Work out the finished part from the listing and answer in its coordinate system (mm). Round coordinates to 2 decimals unless told otherwise and drop trailing zeros. Loops run counter-clockwise (first coordinate to the right, second up) from the corner with the lowest first, then second, coordinate; pieces in that order, holes last.
```python
from build123d import *

# Parameters (mm, degrees)
TD_STD_FEATURE_DEPTH            = 21.0312
ISA_STD_FEATURE_DEPTH           = 22.061040395498036
ISA_STD_FEATURE_DEPTH_BACK      = 22.061040395498036
BA_STD_FEATURE_DEPTH            = 22.061040395498036
BA_STD_FEATURE_DEPTH_BACK       = 22.061040395498036
VR_STD_FEATURE_DEPTH            = 22.061040395498036
VR_STD_FEATURE_DEPTH_BACK       = 22.061040395498036
ND_STD_FEATURE_DEPTH            = 22.061040395498036
ND_STD_FEATURE_DEPTH_BACK       = 22.061040395498036
HOLE_STD_FEATURE_D              = 0.381
HOLE_STD_FEATURE_CSINK_D        = 0.635
HOLE_STD_FEATURE_CSINK_ANGLE    = 60
STD_HOLE_CUT_FEATURE_DEPTH      = 22.158574025318714
STD_HOLE_CUT_FEATURE_DEPTH_BACK = 22.158574025318714
NR_FEATURE_R                    = 0.0254
STD_C_FEATURE_DEPTH             = 22.061040395498036
STD_C_FEATURE_DEPTH_BACK        = 22.061040395498036
STD_FR_C_FEATURE_R              = 0.01016
STD_BR_C_FEATURE_R              = 0.01016


with BuildPart() as part:
    # td_std_sketch → td_std_feature (new body)
    with BuildSketch(Plane(origin=(0, 0, 0), x_dir=(1, 0, 0), z_dir=(0, 1, 0))):
        with BuildLine():
            Line((-0.65532, 0.4456234374446657), (-0.6553199999999998, -0.44562343744466604))
            ThreePointArc((-0.6553199999999998, -0.44562343744466604), (0.79248, 0), (-0.65532, 0.4456234374446657))
        make_face()
    extrude(amount=TD_STD_FEATURE_DEPTH)

    # isa_std_sketch → isa_std_feature (cut, two sides: drawn at the far end of the back side and taken through both)
    with BuildSketch(Plane(origin=(0, 0, 0), x_dir=(0, 0, -1), z_dir=(1, 0, 0)).offset(-ISA_STD_FEATURE_DEPTH_BACK)):
        Polygon((8.373162888528082, 47.27049062508045), (0.79248, 4.278301579083286), (0.03809999999999999, 0), (-0.03809999999999999, 0), (-0.79248, 4.278301579083286), (-8.373162888528082, 47.27049062508045), (-8.373162888528082, -40.04033509597618), (8.373162888528082, -40.04033509597618), align=None)
    extrude(amount=ISA_STD_FEATURE_DEPTH + ISA_STD_FEATURE_DEPTH_BACK, mode=Mode.SUBTRACT)

    # ba_std_sketch → ba_std_feature (cut, two sides: drawn at the far end of the back side and taken through both)
    with BuildSketch(Plane.XY.offset(-BA_STD_FEATURE_DEPTH_BACK)):
        Polygon((-51.96869655836785, -9.056666233848073), (-0.6057899999999999, 0), (-0.4471889008518133, 0.02796565294984382), (0.79248, 7.0584773526961735), (9.849146233848053, 58.421383911064034), (86.76310584868799, -12.040863498073982), (24.945263056472086, -79.51891364298609), align=None)
    extrude(amount=BA_STD_FEATURE_DEPTH + BA_STD_FEATURE_DEPTH_BACK, mode=Mode.SUBTRACT)

    # vr_std_sketch → vr_std_feature (cut, two sides: drawn at the far end of the back side and taken through both)
    with BuildSketch(Plane(origin=(0, 0, 0), x_dir=(0, 0, -1), z_dir=(1, 0, 0)).offset(-VR_STD_FEATURE_DEPTH_BACK)):
        with BuildLine():
            Line((35.91518958962539, 36.381828135911775), (0.79248, 1.2591185462865075))
            Line((0.79248, 1.2591185462865075), (0.24587123921628848, 0.7125097855027981))
            ThreePointArc((0.24587123921628848, 0.7125097855027981), (0.14656815960932523, 0.5719991778386461), (0.09986436121197133, 0.40640000000000004))
            Line((0.09986436121197133, 0.40640000000000004), (0.05714999999999999, 0))
            Line((0.05714999999999999, 0), (-0.05714999999999999, 0))
            Line((-0.05714999999999999, 0), (-0.09986436121197133, 0.40640000000000004))
            ThreePointArc((-0.09986436121197133, 0.40640000000000004), (-0.14656815960932523, 0.5719991778386461), (-0.24587123921628848, 0.7125097855027981))
            Line((-0.24587123921628848, 0.7125097855027981), (-0.79248, 1.2591185462865075))
            Line((-0.79248, 1.2591185462865075), (-35.91518958962539, 36.381828135911775))
            Line((-35.91518958962539, 36.381828135911775), (-35.91518958962539, -62.96019636196763))
            Line((-35.91518958962539, -62.96019636196763), (35.91518958962539, -62.96019636196763))
            Line((35.91518958962539, -62.96019636196763), (35.91518958962539, 36.381828135911775))
        make_face()
    extrude(amount=VR_STD_FEATURE_DEPTH + VR_STD_FEATURE_DEPTH_BACK, mode=Mode.SUBTRACT)

    # nd_std_sketch → nd_std_feature (cut, two sides: drawn at the far end of the back side and taken through both)
    with BuildSketch(Plane.XY.offset(-ND_STD_FEATURE_DEPTH_BACK)):
        Polygon((-26.695612432299043, -45.16910067246157), (-0.6172199999999999, 0), (-0.5795900153763918, 0.06517704525612475), (-0.49309651581291747, 0.01523999999999999), (44.67600415664865, -26.06315243229904), (71.65060635143378, -126.82868059585769), (0.27898976248608776, -145.93462883602024), align=None)
    extrude(amount=ND_STD_FEATURE_DEPTH + ND_STD_FEATURE_DEPTH_BACK, mode=Mode.SUBTRACT)

    # hole_std_feature (through all)
    with Locations(Plane(origin=(0, 21.0312, 0), x_dir=(1, 0, 0), z_dir=(0, 1, 0))):
        with Locations((0, 0)):
            CounterSinkHole(HOLE_STD_FEATURE_D / 2, HOLE_STD_FEATURE_CSINK_D / 2, counter_sink_angle=HOLE_STD_FEATURE_CSINK_ANGLE)


with BuildPart() as body_2:
    # std_hole_sketch → std_hole_feature (revolve)
    with BuildSketch(Plane.XY):
        Polygon((2.0643967957346323, 1.16621487026174), (1.318693364519402, 1.9119183014769674), (-0.6066953211391621, -0.01347038418160373), (-0.5932249369575584, -0.02694076836320745), (-0.43560320426536, 0.13068096432899157), align=None)
    revolve(axis=Axis((-0.6066953211391621, -0.01347038418160373, 0), (0.7071067811865462, 0.7071067811865488, 0)))

    # std_hole_cut_sketch → std_hole_cut_feature (cut, two sides: drawn at the far end of the back side and taken through both)
    with BuildSketch(Plane.XY.offset(-STD_HOLE_CUT_FEATURE_DEPTH_BACK)):
        Polygon((-45.98482601113434, 26.27990227002553), (-0.6553199999999999, 0.1088997722642913), (-0.557592970120267, 0.05247704525612475), (-0.49309651581291747, 0.01523999999999999), (44.83640949532142, -26.155762497761245), (-7.505595500201061, -116.81477452002991), (-98.32683100665682, -64.37910975224314), align=None)
    extrude(amount=STD_HOLE_CUT_FEATURE_DEPTH + STD_HOLE_CUT_FEATURE_DEPTH_BACK, mode=Mode.SUBTRACT)


with BuildPart() as part_1:
    add(part.part)

    # std_hole_combine: cut body 2
    add(body_2.part, mode=Mode.SUBTRACT)

    # nr_feature
    nr_feature_edges = [part_1.edges().sort_by_distance(p)[0] for p in [
        (-0.5795900153763918, 0.06517704525612475, 0),
    ]]
    fillet(nr_feature_edges, radius=NR_FEATURE_R)

    # std_c_sketch → std_c_feature (cut, two sides: drawn at the far end of the back side and taken through both)
    with BuildSketch(Plane(origin=(0, 0, 0), x_dir=(0, 0, -1), z_dir=(1, 0, 0)).offset(-STD_C_FEATURE_DEPTH_BACK)):
        with BuildLine():
            Line((51.47071118925243, -8.282224024034191), (0.03810000000000001, -3e-17))
            ThreePointArc((0.03810000000000001, -3e-17), (1e-17, 0.00304799999999997), (-0.03809999999999998, -3e-17))
            Line((-0.03809999999999998, -3e-17), (-51.47071118925243, -8.282224024034191))
            Line((-51.47071118925243, -8.282224024034191), (-51.47071118925243, -112.47260224638451))
            Line((-51.47071118925243, -112.47260224638451), (51.47071118925243, -112.47260224638451))
            Line((51.47071118925243, -112.47260224638451), (51.47071118925243, -8.282224024034191))
        make_face()
    extrude(amount=STD_C_FEATURE_DEPTH + STD_C_FEATURE_DEPTH_BACK, mode=Mode.SUBTRACT)

    # std_fr_c_feature
    std_fr_c_feature_edges = [part_1.edges().sort_by_distance(p)[0] for p in [
        (-0.6553199999999999, 0.003048, 7e-17),
    ]]
    fillet(std_fr_c_feature_edges, radius=STD_FR_C_FEATURE_R)

    # std_br_c_feature
    std_br_c_feature_edges = [part_1.edges().sort_by_distance(p)[0] for p in [
        (-0.6154602363795091, 0.00304799999999997, 2e-17),
    ]]
    fillet(std_br_c_feature_edges, radius=STD_BR_C_FEATURE_R)


solid = part_1.part
```
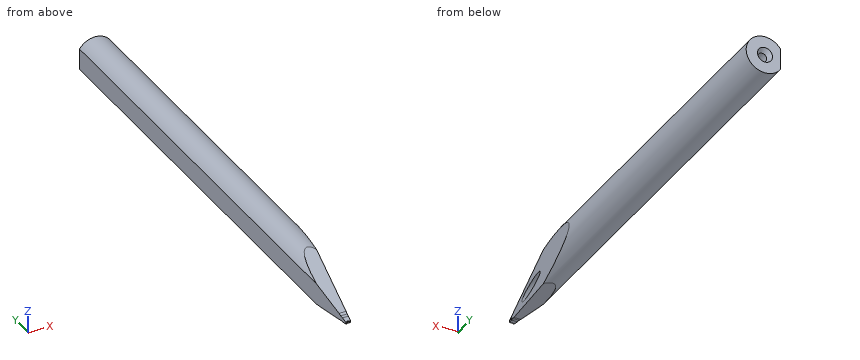
1. Find section A-A (x = 0). Write down the section's boundary in (y, z).
Answer key:
outline: (2.56, -0.49) - (4.28, -0.79) - (21.03, -0.79) - (21.03, -0.32) - (20.81, -0.19) - (2.56, -0.19) - close; (2.56, 0.19) - (20.81, 0.19) - (21.03, 0.32) - (21.03, 0.79) - (4.28, 0.79) - (2.56, 0.49) - close
2. Find section C-C (y = 14.5). Write down the section's boundary in (x, z), then the cut area to 3 significant figures.
Answer key:
outline: (-0.66, -0.45) arc R0.79 ccw (long way) to (-0.66, 0.45) - close; hole circle Ø0.38 at (0, 0)
area: 1.78 mm2
3. Find section B-B (y = 5.75). Write down the section's boundary in (x, z), then the cut area to 3 significant figures.
Answer key:
outline: (-0.66, -0.45) arc R0.79 ccw to (0.56, -0.56) - (0.56, 0.56) arc R0.79 ccw to (-0.66, 0.45) - close; hole circle Ø0.38 at (0, 0)
area: 1.60 mm2
4. Consider probe 1 along Z at (x, y) = (0, 12.5); probe 2 along X at (y, z) = (16.5, -0.05); probe 3 along X at (y, z) = (16.5, -0.3). Determine where each line is inside the solid, lowest interval first.
Answer key:
probe 1: z = -0.79 to -0.19, 0.19 to 0.79
probe 2: x = -0.66 to -0.18, 0.18 to 0.79
probe 3: x = -0.66 to 0.73
